from build123d import *
from OCP.BRepFilletAPI import BRepFilletAPI_MakeChamfer
from build123d.topology import SkipClean

# Parameters (mm, degrees)
EXTRUDE_1_DEPTH      = 2
EXTRUDE_START        = 1.5
SKETCH_2_R           = 3.5
EXTRUDE_2_DEPTH      = 1.5
SKETCH_3_R           = 2.6
CUT_EXTRUDE_1_DEPTH  = 2.5
SKETCH_4_R           = 3.5
EXTRUDE_3_DEPTH      = 1.25
SKETCH_5_R           = 2.5
CUT_EXTRUDE_2_DEPTH  = 1.25
SKETCH_6_R           = 1.25
CUT_EXTRUDE_3_DEPTH  = 19.957584234
EXTRUDE_4_REACH      = 16.132
EXTRUDE_4_END_RADIUS = 3.5
SKETCH_8_W           = 1
SKETCH_8_H           = 1.25
EXTRUDE_5_DEPTH      = 1.25
CHAMFER_2_SIZE       = 1.25
CHAMFER_2_SIZE_2     = 1.5
SKETCH_10_R          = 0.75
CUT_EXTRUDE_4_DEPTH  = 19.957584234


with BuildPart() as part:
    # 草图1 → 凸台-拉伸1 (new body)
    with BuildSketch(Plane(origin=(0, 0, 0), x_dir=(1, 0, 0), z_dir=(0, 1, 0))):
        with BuildLine():
            Line((0.2625, 3.490142368), (16.1725, 2.293522128))
            ThreePointArc((16.1725, 2.293522128), (18.3, 0), (16.1725, -2.293522128))
            Line((16.1725, -2.293522128), (0.2625, -3.490142368))
            ThreePointArc((0.2625, -3.490142368), (-3.5, 0), (0.2625, 3.490142368))
        make_face()
    extrude(amount=EXTRUDE_1_DEPTH)

    # 草图2 → 凸台-拉伸2 (add)
    with BuildSketch(Plane.XZ.offset(EXTRUDE_START)):
        with Locations(Location((0, 0, 0), (0, 0, 270))):
            Circle(SKETCH_2_R)
    extrude(amount=-EXTRUDE_2_DEPTH)

    # 草图3 → 切除-拉伸1 (cut)
    with BuildSketch(Plane.XZ.offset(1.5)):
        with Locations(Location((0, 0, 0), (0, 0, 270))):
            Circle(SKETCH_3_R)
    extrude(amount=-CUT_EXTRUDE_1_DEPTH, mode=Mode.SUBTRACT)

    # 草图4 → 凸台-拉伸3 (add)
    with SkipClean():  # the faces are left unmerged after this step: merging them gives an invalid solid
        with BuildSketch(Plane(origin=(0, 2, 0), x_dir=(1, 0, 0), z_dir=(0, 1, 0))):
            with Locations(Location((0, 0, 0), (0, 0, 90))):
                Circle(SKETCH_4_R)
        extrude(amount=EXTRUDE_3_DEPTH)

    # 草图5 → 切除-拉伸2 (cut)
    with SkipClean():  # the faces are left unmerged after this step: merging them gives an invalid solid
        with BuildSketch(Plane(origin=(0, 3.25, 0), x_dir=(1, 0, 0), z_dir=(0, 1, 0))):
            with Locations(Location((0, 0, 0), (0, 0, 270))):
                Circle(SKETCH_5_R)
        extrude(amount=-CUT_EXTRUDE_2_DEPTH, mode=Mode.SUBTRACT)

    # 草图6 → 切除-拉伸3 (cut, through all)
    with SkipClean():  # the faces are left unmerged after this step: merging them gives an invalid solid
        with BuildSketch(Plane(origin=(0, 2, 0), x_dir=(1, 0, 0), z_dir=(0, 1, 0))):
            with Locations(Location((0, 0, 0), (0, 0, 270))):
                Circle(SKETCH_6_R)
        extrude(amount=-CUT_EXTRUDE_3_DEPTH, mode=Mode.SUBTRACT)

    # 凸台-拉伸4: up to this cylinder (the profile starts outside it)
    with SkipClean():  # the faces are left unmerged after this step: merging them gives an invalid solid
        extrude_4_end = Plane(origin=(0, 2.625, 0), z_dir=(0, -1, 0)) * Cylinder(EXTRUDE_4_END_RADIUS, 40.264, mode=Mode.PRIVATE)
        # 草图8 → 凸台-拉伸4 (add, up to the surface)
        with BuildSketch(Plane(origin=(5, 0, 0), x_dir=(0, 0, -1), z_dir=(1, 0, 0)), mode=Mode.PRIVATE) as extrude_4_sk1:
            with Locations((0, 2.625)):
                Rectangle(SKETCH_8_W, SKETCH_8_H)
        extrude_4_tool1 = extrude(extrude_4_sk1.sketch, amount=-EXTRUDE_4_REACH, mode=Mode.PRIVATE) - extrude_4_end
        add(extrude_4_tool1.solids().sort_by_distance((5, 2.625, 0))[0])

    # 草图9 → 凸台-拉伸5 (add)
    with SkipClean():  # the faces are left unmerged after this step: merging them gives an invalid solid
        with BuildSketch(Plane(origin=(0, 2, 0), x_dir=(1, 0, 0), z_dir=(0, 1, 0))):
            with BuildLine():
                Line((0.2625, 3.490142368), (5, 3.133826316))
                Line((5, 3.133826316), (5, 2.133826316))
                Line((5, 2.133826316), (2.627432324, 2.312271476))
                ThreePointArc((2.627432324, 2.312271476), (1.56037565, 3.1329264), (0.2625, 3.490142368))
            make_face()
            with BuildLine():
                Line((0.2625, -3.490142368), (5, -3.133826316))
                Line((5, -3.133826316), (5, -2.133826316))
                Line((5, -2.133826316), (2.627432324, -2.312271476))
                ThreePointArc((2.627432324, -2.312271476), (1.56037565, -3.1329264), (0.2625, -3.490142368))
            make_face()
        extrude(amount=EXTRUDE_5_DEPTH)

    # 倒角2
    chamfer_2_edges_1 = [part.edges().sort_by_distance(p)[0] for p in [
        (5, 3.25, 2.633826316),
    ]]
    chamfer_2_side_1 = [part.faces().sort_by_distance(p)[0] for p in [
        (5, 3.225, 2.633826316),
    ]]
    chamfer_2_edges_2 = [part.edges().sort_by_distance(p)[0] for p in [
        (5, 3.25, -2.633826316),
    ]]
    chamfer_2_side_2 = [part.faces().sort_by_distance(p)[0] for p in [
        (5, 3.225, -2.633826316),
    ]]
    chamfer_2_edges_3 = [part.edges().sort_by_distance(p)[0] for p in [
        (5, 3.25, 0),
    ]]
    chamfer_2_side_3 = [part.faces().sort_by_distance(p)[0] for p in [
        (5, 3.225, 0),
    ]]
    chamfer_2 = BRepFilletAPI_MakeChamfer(part.part.solid().wrapped)
    for e in chamfer_2_edges_1:
        chamfer_2.Add(CHAMFER_2_SIZE - 0.0001, CHAMFER_2_SIZE_2 - 0.0001, e.wrapped, chamfer_2_side_1[0].wrapped)
    for e in chamfer_2_edges_2:
        chamfer_2.Add(CHAMFER_2_SIZE - 0.0001, CHAMFER_2_SIZE_2 - 0.0001, e.wrapped, chamfer_2_side_2[0].wrapped)
    for e in chamfer_2_edges_3:
        chamfer_2.Add(CHAMFER_2_SIZE - 0.0001, CHAMFER_2_SIZE_2 - 0.0001, e.wrapped, chamfer_2_side_3[0].wrapped)
    add(Compound.cast(chamfer_2.Shape()), mode=Mode.REPLACE)  # a hair under: the kernel refuses the full size

    # 草图10 → 切除-拉伸4 (cut, through all)
    with BuildSketch(Plane(origin=(0, 2, 0), x_dir=(1, 0, 0), z_dir=(0, 1, 0))):
        with Locations(Location((5.75, 0, 0), (0, 0, 270))):
            Circle(SKETCH_10_R)
        with Locations(Location((8.3125, 0, 0), (0, 0, 270))):
            Circle(SKETCH_10_R)
        with Locations(Location((10.875, 0, 0), (0, 0, 270))):
            Circle(SKETCH_10_R)
        with Locations(Location((13.4375, 0, 0), (0, 0, 270))):
            Circle(SKETCH_10_R)
        with Locations(Location((16, 0, 0), (0, 0, 270))):
            Circle(SKETCH_10_R)
    extrude(amount=-CUT_EXTRUDE_4_DEPTH, mode=Mode.SUBTRACT)


solid = part.part
Work out the finished part from the listing and answer in its coordinate system (mm). A direction names the side the tool comes from. Round coordinates to 2 decimals unless told otherwise and drop trailing zeros. Loops run counter-clockwise (first coordinate to the right, second up) from the corner with the lowest first, then second, coordinate; pieces in that order, holes last. Notation, with made-up numbers: (29.25, 75.5) - (35.25, 75.5) arc R26 cw to (35.25, 95.5) - close; hole circle Ø1 at (71.25, 78). An arc over 180 degrees is marked (long way). Use one line per item in the form item = value. Start each with the question number.
(1) Which of the six approach directions +Z, -Z, +X, -X, +Y, -Y give full straight-line access (tool end or side, diameter ignored) to faces 1 (the face through (4.1, 2.5, -0.5)), 2 (the face through (0.78, -0.27, -2.48)), 3 (the face through (1, 2, 1))?
(2) Find section D-D on x = 6.25. Determine the outline of the cut face in (y, z).
(3) Find section A-A on x = 0. Determine the outline of the cut face in (y, z), and give its area (3 significant figures).
(4) Consider line 1 (Y direction, x = 15.75, z = 2); line 2 (X direction, y = 1.45, z = 1); line 3 (Z direction, x = 13.25, y = 1.3). Determine where each line is inside the solid, lowest interval first.
(5) Determine the mould class of faces 4 (the face through (15.268, 1.014, -0.163)), 5 (the face through (3, -1.5, 0)), 6 (the face through (4.24, 2.634, 0.007)) for opening direction X: +X half, -X half, draft (parallel to the pull), parting line (faces both ways), or undercut.
(6) Find section B-B on z = 1. Determine the outline of the cut face in (x, y), and give its area (3 significant figures).
(7) Flat-ended cylindrical pins translate along their axes: P1, Ø1.7, axis at x = 5.75, z = 0, coming from the +Y side; P2, Ø1.7, axis at x = 16, z = 0, coming from the +Y side; P3, Ø3.5, axis at x = 7.5, z = -1.5, coming from the -Y side; P4, Ø1.4, axis at x = 13.44, z = 0, coming from the -Y side. Find the tip coordinate at first contact, or state that the pin passes through.
(8) Find section C-C on y = 1.6. Give the number of separate pieces and of enclosed holes in the cut face, and give its area (3 significant figures).
Answer list:
q1.face_1 = +X, +Y
q1.face_2 = -Y
q1.face_3 = +Y
q2.outline = (0, -3.04) - (2, -3.04) - (2, -0.56) - (0, -0.56) - close; (0, 0.56) - (2, 0.56) - (2, 3.04) - (0, 3.04) - close
q3.outline = (-1.5, -3.5) - (3.25, -3.5) - (3.25, -2.5) - (2, -2.5) - (2, -1.25) - (1, -1.25) - (1, -2.6) - (-1.5, -2.6) - close; (-1.5, 2.6) - (1, 2.6) - (1, 1.25) - (2, 1.25) - (2, 2.5) - (3.25, 2.5) - (3.25, 3.5) - (-1.5, 3.5) - close
q3.area = 11.5 mm^2
q4.line_1 = 0 to 2
q4.line_2 = -3.35 to -0.75, 0.75 to 18.07
q4.line_3 = -2.51 to -0.73, 0.73 to 2.51
q5.face_4 = undercut
q5.face_5 = draft
q5.face_6 = +X half
q6.outline = (-3.35, -1.5) - (-2.4, -1.5) - (-2.4, 1) - (-0.75, 1) - (-0.75, 2) - (-2.29, 2) - (-2.29, 3.25) - (-3.35, 3.25) - close; (0.75, 1) - (2.4, 1) - (2.4, -1.5) - (3.35, -1.5) - (3.35, 0) - (18.07, 0) - (18.07, 2) - (3.35, 2) - (3.35, 3.25) - (2.29, 3.25) - (2.29, 2) - (0.75, 2) - close
q6.area = 42.1 mm^2
q7.P1 = 2.08
q7.P2 = 2
q7.P3 = 0
q7.P4 = through
q8.separate_pieces = 1
q8.enclosed_holes = 6
q8.area = 107 mm^2
